from build123d import *

# Parameters (mm, degrees)
SKETCH1_R              = 52
BOSS_EXTRUDE1_DEPTH    = 25
CUT_EXTRUDE1_DEPTH     = 25
SKETCH3_R              = 6.5
CUT_EXTRUDE2_DEPTH     = 30
SKETCH5_R              = 6.5
CUT_EXTRUDE3_DEPTH     = 30
SKETCH6_W              = 13
SKETCH6_H              = 90.106241662
SKETCH6_H_2            = 26.210700472
SKETCH6_H_3            = 29.761182449
CUT_EXTRUDE4_DEPTH     = 30
M3_TAPPED_HOLE1_REACH  = 120.933
M3_TAPPED_HOLE1_BORE_R = 1.25
SKETCH10_R             = 5
CUT_EXTRUDE5_DEPTH     = 30


with BuildPart() as part:
    # Sketch1 → Boss-Extrude1 (new body)
    with BuildSketch(Plane.XY):
        Circle(SKETCH1_R)
    extrude(amount=BOSS_EXTRUDE1_DEPTH)

    # Sketch2 → Cut-Extrude1 (cut)
    with BuildSketch(Plane.XY.offset(25)):
        with BuildLine():
            Line((32, 0), (32, -45))
            Line((32, -45), (42, -45))
            Line((42, -45), (42, 3.54e-07))
            ThreePointArc((42, 3.54e-07), (36.999999823, 5), (32, 0))
        make_face()
        with BuildLine():
            Line((-5, -39.999999646), (-5, -55))
            Line((-5, -55), (5, -55))
            Line((5, -55), (5, -40))
            ThreePointArc((5, -40), (1.77e-07, -35), (-5, -39.999999646))
        make_face()
        with BuildLine():
            Line((-32, -45), (-42, -45))
            Line((-42, -45), (-42, 3.54e-07))
            ThreePointArc((-42, 3.54e-07), (-36.999999823, 5), (-32, 0))
            Line((-32, 0), (-32, -45))
        make_face()
    extrude(amount=-CUT_EXTRUDE1_DEPTH, mode=Mode.SUBTRACT)

    # Sketch3 → Cut-Extrude2 (cut)
    with BuildSketch(Plane.XY.offset(25)):
        with Locations((0, 34)):
            Circle(SKETCH3_R)
    extrude(amount=-CUT_EXTRUDE2_DEPTH, mode=Mode.SUBTRACT)

    # Sketch5 → Cut-Extrude3 (cut)
    with BuildSketch(Plane.XY.offset(25)):
        with Locations((-24.04163056, -24.04163056)):
            Circle(SKETCH5_R)
    cut_extrude3 = extrude(amount=-CUT_EXTRUDE3_DEPTH, mode=Mode.SUBTRACT)

    # Mirror1: Cut-Extrude3 across plane
    add(cut_extrude3.mirror(Plane(origin=(0, 0, 0), x_dir=(0, 0, 1), z_dir=(1, 0, 0))), mode=Mode.SUBTRACT)

    # Sketch6 → Cut-Extrude4 (cut)
    with BuildSketch(Plane.XY.offset(25)):
        with Locations((0, -11.053120831)):
            Rectangle(SKETCH6_W, SKETCH6_H)
        with Locations((24.04163056, -37.146980796)):
            Rectangle(SKETCH6_W, SKETCH6_H_2)
        with Locations((-24.04163056, -38.922221785)):
            Rectangle(SKETCH6_W, SKETCH6_H_3)
    extrude(amount=-CUT_EXTRUDE4_DEPTH, mode=Mode.SUBTRACT)

    # M3 Tapped Hole1 bore → M3 Tapped Hole1 (cut, up to next)
    with BuildSketch(Plane.ZY.offset(52), mode=Mode.PRIVATE) as m3_tapped_hole1_sk1:
        with Locations((12.5, 0)):
            Circle(M3_TAPPED_HOLE1_BORE_R)
    m3_tapped_hole1_tool1 = extrude(m3_tapped_hole1_sk1.sketch, amount=-M3_TAPPED_HOLE1_REACH, mode=Mode.PRIVATE) & part.part
    m3_tapped_hole1 = m3_tapped_hole1_tool1.solids().sort_by_distance((-52, 0, 12.5))[0]
    add(m3_tapped_hole1, mode=Mode.SUBTRACT)

    # Mirror2: M3 Tapped Hole1 across plane
    add(m3_tapped_hole1.mirror(Plane(origin=(0, 0, 0), x_dir=(0, 0, 1), z_dir=(1, 0, 0))), mode=Mode.SUBTRACT)

    # Sketch10 → Cut-Extrude5 (cut)
    with BuildSketch(Plane.XY.offset(25)):
        with Locations((28.284271247, 28.284271247)):
            Circle(SKETCH10_R)
    cut_extrude5 = extrude(amount=-CUT_EXTRUDE5_DEPTH, mode=Mode.SUBTRACT)

    # Mirror3: Cut-Extrude5 across plane
    add(cut_extrude5.mirror(Plane(origin=(0, 0, 0), x_dir=(0, 0, 1), z_dir=(1, 0, 0))), mode=Mode.SUBTRACT)


solid = part.part
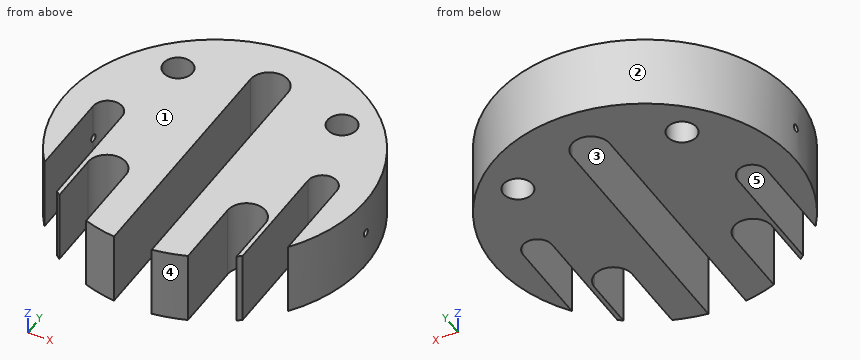
Here's how the part is built. I have some questions about the finished solid (model axes, mm). Face numbers are marked on the shaded views. A direction names the side the tool comes from. Give positions to 0.01 mm unless a question says otherwise; leave off trailing zeros. Write each loop counter-clockwise with the first axis right and the second up, starting at its lowest first coordinate (ties: lowest second). Pieces come first, ordered by that corner, then holes. Notation, with made-up numbers: (13.5, 33) -> (59.5, 33) arc R23 ccw to (59.5, 62) -> close; hole circle Ø10 at (-18, 26). An arc over 180 degrees is marked (long way). Use one line per item in the form item = value. Start each with the question number.
1. Imagine slicing it at C-C on x = 0. List the corners of the cut face in (y, z) for me, plus the area to 4 significant figures.
2. If I drill on L1, parallel to X at y = -38.5, z = 3.5; L2, parallel to X at y = -22, z = 4; L3, parallel to X at y = -46.5, z = 12, over which ranges is the centre line in solid material (lowest first)?
3. Thinking about a two-plate mould opening in X: for the marked faces 1, 2 and 3, which applies, +X half, -X half, draft (parallel to the pull), parting line (faces both ways), or undercut?
4. Imagine slicing it at B-B on y = -29. List the corners of the cut face in (x, z) for me.
5. On a 3-axis mill with a long thin cutter (end or side, diameter ignored), from which of +Z, -Z, +X, -X, +Y, -Y can I reach the whole of each face in a straight line? I mean the marked faces 4 and 5. Say none if no direction works.
6. Imagine slicing it at A-A on z = 15.25. List the corners of the cut face in (x, y) for me, plus the area to 3 significant figures.
7. Will these pins go through, and if not, where does the flat tip stop? pin 1 Ø1 at (x, y) = (-23, -19.5) entering from +Z; pin 2 Ø2 at (y, z) = (0, 12.5) entering from +X; pin 3 Ø10 at (y, z) = (14.5, 5) entering from -X; pin 4 Ø7.5 at (y, z) = (-14, 7) entering from -X.
8. Imagine slicing it at D-D on x = -37. List the corners of the cut face in (y, z) for me.
Entries:
q1.outline = (40.5, 0) -> (52, 0) -> (52, 25) -> (40.5, 25) -> close
q1.area = 287.5 mm²
q2.L1 = -32 to -30.54, -17.54 to -6.5, 6.5 to 17.54, 30.54 to 32
q2.L2 = -47.12 to -42, -32 to -30.21, -17.87 to -6.5, 6.5 to 17.87, 30.21 to 32, 42 to 47.12
q2.L3 = -17.54 to -6.5, 6.5 to 17.54
q3.face_1 = draft
q3.face_2 = parting line
q3.face_3 = undercut
q4.outline = (-43.16, 0) -> (-42, 0) -> (-42, 25) -> (-43.16, 25) -> close; (-32, 0) -> (-30.54, 0) -> (-30.54, 25) -> (-32, 25) -> close; (-17.54, 0) -> (-6.5, 0) -> (-6.5, 25) -> (-17.54, 25) -> close; (6.5, 0) -> (17.54, 0) -> (17.54, 25) -> (6.5, 25) -> close; (30.54, 0) -> (32, 0) -> (32, 25) -> (30.54, 25) -> close; (42, 0) -> (43.16, 0) -> (43.16, 25) -> (42, 25) -> close
q5.face_4 = +Z, -Z, +X, -Y
q5.face_5 = +Z, -Z, -Y
q6.outline = (-42, -30.66) -> (-42, 0) arc R5 cw to (-32, 0) -> (-32, -40.99) arc R52 ccw to (-30.54, -42.09) -> (-30.54, -24.04) arc R6.5 cw to (-17.54, -24.04) -> (-17.54, -48.95) arc R52 ccw to (-6.5, -51.59) -> (-6.5, 34) arc R6.5 cw to (6.5, 34) -> (6.5, -51.59) arc R52 ccw to (17.54, -48.95) -> (17.54, -24.04) arc R6.5 cw to (30.54, -24.04) -> (30.54, -42.09) arc R52 ccw to (32, -40.99) -> (32, 0) arc R5 cw to (42, 0) -> (42, -30.66) arc R52 ccw (long way) to start; hole circle Ø10 at (-28.28, 28.28); hole circle Ø10 at (28.28, 28.28)
q6.area = 5,650 mm²
q7.pin_1 = through
q7.pin_2 = 32.1
q7.pin_3 = -51.12
q7.pin_4 = -50.98
q8.outline = (5, 0) -> (36.54, 0) -> (36.54, 25) -> (5, 25) -> close
